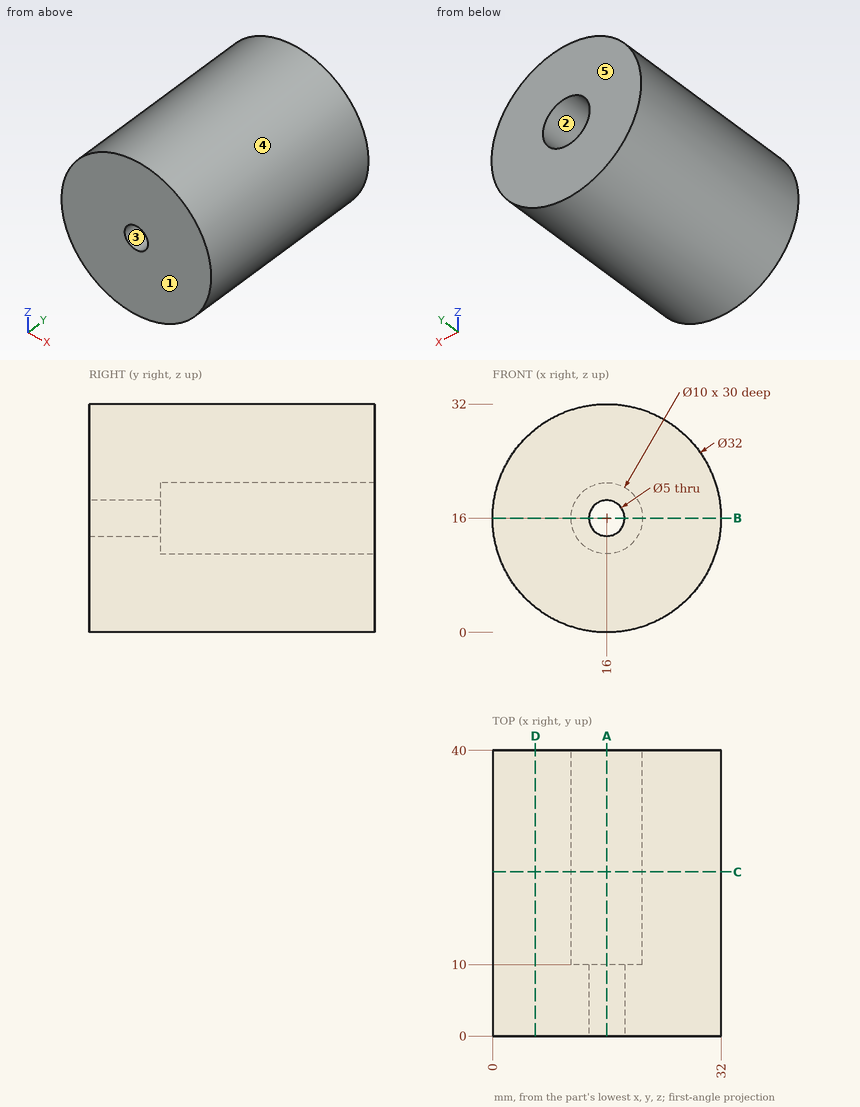
Print and shaded views of the part. All mm, measured from the part's lowest x, y and z. A direction names the side the tool comes from. Give positions to 0.01 mm unless a question says otherwise; leave off trailing zeros. Loops run counter-clockwise (first coordinate to the right, second up) from the corner with the lowest first, then second, coordinate; pieces in that order, holes last.
1) Saw through at C-C (y = 23). Write the cut outline in (x, z).
2) Flat gauge pins, fed straight in: pin 1 Ø11.5 at (x, z) = (16, 16) entering from -Y; pin 2 Ø10 at (x, y) = (4.5, 23.5) entering from +Z; pin 3 Ø3 at (x, y) = (18.5, 19) entering from +Z; pin 4 Ø2 at (x, y) = (24.5, 19) entering from -Z. Where does each tip first touch, or does it go through?
3) Saw through at B-B (z = 16). Write the cut outline in (x, y), plus the area to 3 significant figures.
4) Saw through at D-D (x = 6). Write the cut outline in (y, z), plus the area to 3 significant figures.
5) Wall check: line 1 (X direction, y = 26.5, z = 16); line 2 (X direction, y = 2.5, z = 16); line 3 (Y direction, x = 17.5, z = 13.5). Give the ranges that are in metal, low to high.
6) Pull direction Z, two halves, no side cores. Call the marked faces 3, 4 and 5: +Z half, -Z half, draft (parallel to the pull), parting line (faces both ways), or undercut.
7) Tool access for the marked faces 1 and 2: list every direction of +Z, -Z, +X, -X, +Y, -Y with a clear straight run to the whole face (end or side of a thin tool).
8) Saw through at A-A (x = 16). Write the cut outline in (y, z).
Answer block:
1. outline: circle Ø32 at (16, 16); hole circle Ø10 at (16, 16)
2. pin 1: stops at y = 0
2. pin 2: stops at z = 30.62
2. pin 3: stops at z = 31.97
2. pin 4: stops at z = 1.87
3. outline: (0, 0) - (13.5, 0) - (13.5, 10) - (11, 10) - (11, 40) - (0, 40) - close; (18.5, 0) - (32, 0) - (32, 40) - (21, 40) - (21, 10) - (18.5, 10) - close
3. area: 930 mm2
4. outline: (0, 3.51) - (40, 3.51) - (40, 28.49) - (0, 28.49) - close
4. area: 999 mm2
5. line 1: x = 0 to 11, 21 to 32
5. line 2: x = 0 to 13.5, 18.5 to 32
5. line 3: y = 0 to 10
6. face 3: undercut
6. face 4: parting line
6. face 5: draft
7. face 1: +Z, -Z, +X, -X, -Y
7. face 2: +Y
8. outline: (0, 0) - (40, 0) - (40, 11) - (10, 11) - (10, 13.5) - (0, 13.5) - close; (0, 18.5) - (10, 18.5) - (10, 21) - (40, 21) - (40, 32) - (0, 32) - close
